Geometry check sheet. Reference: the model listing, model coordinates, mm. Face numbers are marked on the shaded views. A direction names the side the tool comes from. Give positions to 0.01 mm unless a question says otherwise; leave off trailing zeros. Write each loop counter-clockwise with the first axis right and the second up, starting at its lowest first coordinate (ties: lowest second). Pieces come first, ordered by that corner, then holes. Notation, with made-up numbers: (75.25, 85) -> (100.25, 85) arc R13 cw to (100.25, 107) -> close; hole circle Ø5 at (-7.75, -21). An arc over 180 degrees is marked (long way). Write item = value, one per line. Start each with the question number.
1. Depth check by flat-ended pin: P1, Ø4, axis at x = -4.5, z = -6, coming from the -Y side; P2, Ø6, axis at y = 1.5, z = 3.5, coming from the -X side; P3, Ø5, axis at x = -4.5, y = 8, coming from the -Z side. Enter the tip coordinate at first touch or a pass-through.
2. Set-up check for the marked faces 1 and 2: record each of +Z, -Z, +X, -X, +Y, -Y from which the full face is reachable in a straight line by a thin tool's end or side.
3. Cross-section at A-A, the plane y = 6.5. Record the cut outline in (x, z).
4. Cross-section at B-B, the plane y = 3. Record the cut outline in (x, z).
5. Thickness scan on line 1 along Y through (x, z) = (1, -6.75); line 2 along X through (y, z) = (9, 2.25); line 3 along Z through (x, y) = (-5.75, 7.75). Record the ranges inside material, lowest first.
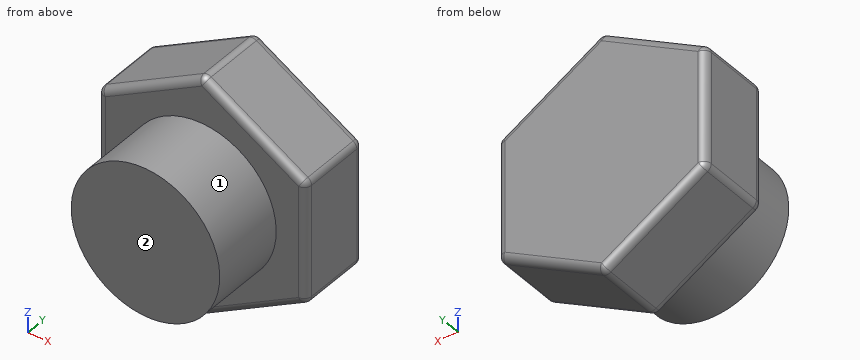
```python
from build123d import *

# Parameters (mm, degrees)
SKETCH1_R           = 5
BOSS_EXTRUDE1_DEPTH = 5
BOSS_EXTRUDE2_DEPTH = 5
FILLET1_R           = 0.5


with BuildPart() as part:
    # Sketch1 → Boss-Extrude1 (new body)
    with BuildSketch(Plane(origin=(0, 0, 0), x_dir=(1, 0, 0), z_dir=(0, 1, 0))):
        with Locations(Location((0, 0, 0), (0, 0, 270))):
            Circle(SKETCH1_R)
    extrude(amount=BOSS_EXTRUDE1_DEPTH)

    # Sketch2 → Boss-Extrude2 (add)
    with BuildSketch(Plane(origin=(0, 5, 0), x_dir=(1, 0, 0), z_dir=(0, 1, 0))):
        Polygon((7.004330674, -4.046297386), (7.006361665, 4.042779607), (0.002030991, 8.089076993), (-7.004330674, 4.046297386), (-7.006361665, -4.042779607), (-0.002030991, -8.089076993), align=None)
    extrude(amount=BOSS_EXTRUDE2_DEPTH)

    # Fillet1
    fillet1_edges = [part.edges().sort_by_distance(p)[0] for p in [
        (3.501149842, 5, 6.06768719),
        (-0.002030991, 7.5, 8.089076993),
        (7.00534617, 5, 0.00175889),
        (7.004330674, 7.5, 4.046297386),
        (3.504196328, 5, -6.0659283),
        (7.006361665, 7.5, -4.042779607),
        (-3.501149842, 5, -6.06768719),
        (0.002030991, 7.5, -8.089076993),
        (-7.00534617, 5, -0.00175889),
        (-7.004330674, 7.5, -4.046297386),
        (-3.504196328, 5, 6.0659283),
        (-7.006361665, 7.5, 4.042779607),
        (3.501149842, 10, 6.06768719),
        (7.00534617, 10, 0.00175889),
        (3.504196328, 10, -6.0659283),
        (-3.501149842, 10, -6.06768719),
        (-7.00534617, 10, -0.00175889),
        (-3.504196328, 10, 6.0659283),
    ]]
    fillet(fillet1_edges, radius=FILLET1_R)


solid = part.part
```
Answers:
q1.P1 = 5
q1.P2 = -4.97
q1.P3 = -6.93
q2.face_1 = -Y
q2.face_2 = +Z, -Z, +X, -X, -Y
q3.outline = (-7.01, 3.75) -> (-7, -3.76) arc R0.5 ccw to (-6.75, -4.19) -> (-0.25, -7.94) arc R0.5 ccw to (0.25, -7.94) -> (6.76, -4.19) arc R0.5 ccw to (7.01, -3.75) -> (7, 3.76) arc R0.5 ccw to (6.75, 4.19) -> (0.25, 7.94) arc R0.5 ccw to (-0.25, 7.94) -> (-6.76, 4.19) arc R0.5 ccw to start
q4.outline = circle Ø10 at (0, 0)
q5.line_1 = 5 to 10
q5.line_2 = -7.01 to 7
q5.line_3 = -4.77 to 4.77
